```python
from build123d import *

# Parameters (mm, degrees)
F0_W      = 23.1
F0_H      = 25.1
F1_DEPTH  = 62.25
F2_W      = 21.1
F2_H      = 60
F3_DEPTH  = 21.1
F4_W      = 3
F4_H      = 1
F5_DEPTH  = 21.1
F6_W      = 4
F6_H      = 30
F7_DEPTH  = 21.1
F9_D      = 2
F9_DEPTH  = 2
F11_D     = 2
F11_DEPTH = 2


with BuildPart() as f1:
    # F0 (on Top) → F1 (new body)
    with BuildSketch(Plane.XY):
        Rectangle(F0_W, F0_H)
    extrude(amount=F1_DEPTH)

    # F2 (on face) → F3 (cut)
    with BuildSketch(Plane.YZ.offset(11.55)):
        with Locations((0, 31.125)):
            Rectangle(F2_W, F2_H)
    extrude(amount=-F3_DEPTH, mode=Mode.SUBTRACT)

    # F4 (on face) → F5 (cut)
    with BuildSketch(Plane.YZ.offset(11.55)):
        with Locations((0, 1.125)):
            Rectangle(F4_W, F4_H)
    extrude(amount=-F5_DEPTH, mode=Mode.SUBTRACT)

    # F6 (on face) → F7 (cut)
    with BuildSketch(Plane.YZ.offset(11.55)):
        with Locations((-12.55, 31.125)):
            Rectangle(F6_W, F6_H)
    extrude(amount=-F7_DEPTH, mode=Mode.SUBTRACT)

    # F9
    with Locations(Plane(origin=(0, 0, 61.125), x_dir=(1, 0, 0), z_dir=(0, 0, -1))):
        with Locations((-8.55, 0)):
            Hole(F9_D / 2, depth=F9_DEPTH)

    # F11
    with Locations(Plane.XY.offset(0.625)):
        with Locations((-8.55, 0)):
            Hole(F11_D / 2, depth=F11_DEPTH)


solid = f1.part
```
Part model, mm, in its own coordinate system. A direction names the side the tool comes from. Round coordinates to 2 decimals unless told otherwise and drop trailing zeros. Write each loop counter-clockwise with the first axis right and the second up, starting at its lowest first coordinate (ties: lowest second). Pieces come first, ordered by that corner, then holes. Notation, with made-up numbers: M 69.5,-20 L 75.5,-20 A15 cw 75.5,-8 Z; hole C 59.25,9.25 d10. An arc over 180 degrees is marked long. One line per question, with ' | ' between items.
(1) Saw through at C-C on y = -7.25. Write the cut outline in (x, z) (3 decimals).
Answer key:
outline: M -11.55,0 L 11.55,0 L 11.55,1.125 L -9.55,1.125 L -9.55,61.125 L 11.55,61.125 L 11.55,62.25 L -11.55,62.25 Z
(2) Pin check, flat tips, straight feed: pin 1 (7 mm diameter, centred on y = -6.5, z = 34.5, fed in from +X); pin 2 (1.8 mm diameter, centred on x = -8.55, y = 0, fed in from +Z); pin 3 (1 mm diameter, centred on x = -3.5, z = 31, fed in from -Y). Stop position of each tip, or through.
Answer key:
pin 1: stops at x = -9.55 | pin 2: passes through | pin 3: stops at y = 10.55
(3) Saw through at A-A on x = -8.55. Write the cut outline in (y, z) (3 decimals), then the cut area to 3 significant figures.
Answer key:
outline: M -12.55,0 L -1,0 L -1,0.625 L -1.5,0.625 L -1.5,1.125 L -10.55,1.125 L -10.55,16.125 L -12.55,16.125 Z; M -12.55,46.125 L -10.55,46.125 L -10.55,61.125 L -1,61.125 L -1,62.25 L -12.55,62.25 Z; M 1,0 L 12.55,0 L 12.55,62.25 L 1,62.25 L 1,61.125 L 10.55,61.125 L 10.55,1.125 L 1.5,1.125 L 1.5,0.625 L 1,0.625 Z | area: 231 mm^2
(4) Saw through at D-D on x = -3.5. Write the cut outline in (y, z) (3 decimals), then the cut area to 3 significant figures.
Answer key:
outline: M -12.55,0 L 12.55,0 L 12.55,62.25 L -12.55,62.25 L -12.55,46.125 L -10.55,46.125 L -10.55,61.125 L 10.55,61.125 L 10.55,1.125 L 1.5,1.125 L 1.5,0.625 L -1.5,0.625 L -1.5,1.125 L -10.55,1.125 L -10.55,16.125 L -12.55,16.125 Z | area: 235 mm^2
(5) Two-plate mould, pull along Y, no slides. Class faces 4 (the face through (0, 12.55, 31)), 5 (the face through (0, 0, 0)), 6 (the face through (-10, -12.55, 31)), 7 (the face through (-9.504, -0.3, 61.695)): released by +Y, released by -Y, zero draft, split by the parting line, or undercut.
Answer key:
face 4: released by +Y | face 5: zero draft | face 6: released by -Y | face 7: undercut
(6) Saw through at B-B on z = 54. Write the cut outline in (x, y).
Answer key:
outline: M -11.55,-12.55 L 11.55,-12.55 L 11.55,-10.55 L -9.55,-10.55 L -9.55,10.55 L 11.55,10.55 L 11.55,12.55 L -11.55,12.55 Z
(7) 3-axis set-ups, long thin cutter, end or side, ignore diameter. For faces 1 (the face through (1, 6, 1.125)), 2 (the face through (1, -12, 46.125)), 3 (the face through (0, 0, 62.25)): which of +Z, -Z, +X, -X, +Y, -Y reach the whole face in a straight line?
Answer key:
face 1: +X | face 2: +X, -Y | face 3: +Z, +X, -X, +Y, -Y
(8) Probe line 1 along Y through (x, z) = (-8.55, 61.95); line 2 along Z through (x, y) = (9.75, -4) (3 decimals); line 3 along Y through (x, z) = (7.25, 10). List the from-to ranges inside material, lowest first.
Answer key:
line 1: y = -12.55 to -1, 1 to 12.55 | line 2: z = 0 to 1.125, 61.125 to 62.25 | line 3: y = -12.55 to -10.55, 10.55 to 12.55
